```python
from build123d import *

# Parameters (mm, degrees)
SKETCH1_W           = 10
SKETCH1_H           = 8
BOSS_EXTRUDE1_DEPTH = 10.9
CHAMFER1_SIZE       = 1.35
CHAMFER1_SIZE2      = 4.0347247
SKETCH2_W           = 10
SKETCH2_H           = 3.5
CUT_EXTRUDE1_DEPTH  = 1.35
SKETCH3_W           = 4
SKETCH3_H           = 5
CUT_EXTRUDE2_DEPTH  = 7
CHAMFER2_SIZE       = 1.2
CUT_EXTRUDE3_DEPTH  = 0.65
SKETCH5_R           = 1.9
CUT_EXTRUDE4_DEPTH  = 5.25
BOSS_EXTRUDE3_DEPTH = 7.4
CUT_EXTRUDE5_DEPTH  = 7.2


with BuildPart() as part:
    # Sketch1 → Boss-Extrude1 (new body)
    with BuildSketch(Plane.XY):
        Rectangle(SKETCH1_W, SKETCH1_H)
    extrude(amount=BOSS_EXTRUDE1_DEPTH)

    # Chamfer1
    chamfer1_edges = [part.edges().sort_by_distance(p)[0] for p in [
        (0, -4, 10.9),
    ]]
    chamfer1_side = [part.faces().sort_by_distance(p)[0] for p in [
        (0, 0, 10.9),
    ]]
    chamfer(chamfer1_edges, length=CHAMFER1_SIZE, length2=CHAMFER1_SIZE2, reference=chamfer1_side[0])

    # Sketch2 → Cut-Extrude1 (cut)
    with BuildSketch(Plane(origin=(0, 4, 0), x_dir=(1, 0, 0), z_dir=(0, 1, 0))):
        with Locations((0, -9.15)):
            Rectangle(SKETCH2_W, SKETCH2_H)
    extrude(amount=-CUT_EXTRUDE1_DEPTH, mode=Mode.SUBTRACT)

    # Sketch3 → Cut-Extrude2 (cut)
    with BuildSketch(Plane.XZ.offset(4)):
        with Locations((-2.475, 3.15)):
            Rectangle(SKETCH3_W, SKETCH3_H)
        with Locations((2.475, 3.15)):
            Rectangle(SKETCH3_W, SKETCH3_H)
    extrude(amount=-CUT_EXTRUDE2_DEPTH, mode=Mode.SUBTRACT)

    # Chamfer2
    chamfer2_edges = [part.edges().sort_by_distance(p)[0] for p in [
        (-2.475, -4, 5.65),
        (2.475, -4, 5.65),
    ]]
    chamfer(chamfer2_edges, length=CHAMFER2_SIZE)

    # Sketch4 → Cut-Extrude3 (cut)
    with BuildSketch(Plane(origin=(0, 0, 0), x_dir=(-1, 0, 0), z_dir=(0, 0, -1))):
        Polygon((2, 0.7), (3, 0.7), (3, -2.4), (3.25, -4), (1.75, -4), (2, -2.4), align=None)
        Polygon((-2, 0.7), (-2, -2.4), (-1.75, -4), (-3.25, -4), (-3, -2.4), (-3, 0.7), align=None)
    extrude(amount=-CUT_EXTRUDE3_DEPTH, mode=Mode.SUBTRACT)

    # Sketch5 → Cut-Extrude4 (cut)
    with BuildSketch(Plane.XY.offset(10.9)):
        with Locations((-2.5, 0)):
            Circle(SKETCH5_R)
        with Locations((2.5, 0)):
            Circle(SKETCH5_R)
    extrude(amount=-CUT_EXTRUDE4_DEPTH, mode=Mode.SUBTRACT)

    # Sketch6 → Boss-Extrude3 (add)
    with BuildSketch(Plane(origin=(0, 0, 0), x_dir=(-1, 0, 0), z_dir=(0, 0, -1))):
        Polygon((5, 3.25), (5, 2.85), (5.5, 2.7), (5.5, 3.4), align=None)
    extrude(amount=-BOSS_EXTRUDE3_DEPTH)

    # Sketch7 → Cut-Extrude5 (cut)
    with BuildSketch(Plane(origin=(0, 0, 0), x_dir=(-1, 0, 0), z_dir=(0, 0, -1))):
        Polygon((-5, 3.25), (-4.5, 3.4), (-4.5, 2.7), (-5, 2.85), align=None)
    extrude(amount=-CUT_EXTRUDE5_DEPTH, mode=Mode.SUBTRACT)


solid = part.part
```
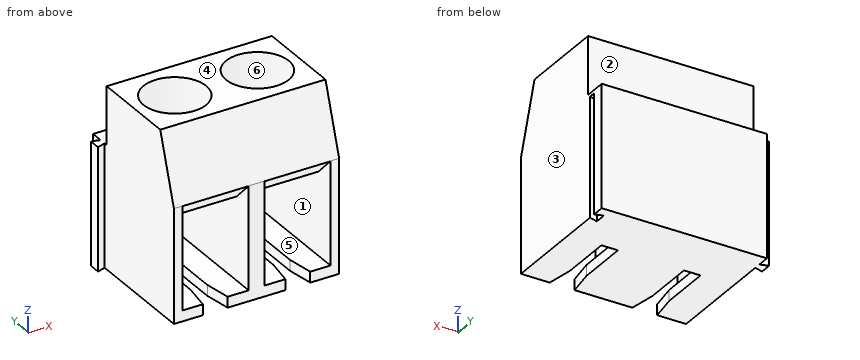
Verification items for the finished model (mm, model axes). Face numbers are marked on the shaded views. A direction names the side the tool comes from. Give positions to 0.01 mm unless a question says otherwise; leave off trailing zeros. Order: outer loops, then holes, each group sorted by start corner. A loop starts at its lowest first (then second) coordinate and runs counter-clockwise, first axis right, second up. Notation, with made-up numbers: (73.25, 26.25) - (82.25, 26.25) arc R11 ccw to (82.25, 36.25) - close; hole circle Ø7 at (30.5, 20). An arc over 180 degrees is marked (long way). Answer as CSV lines item,"result". Start each with the question number.
Item 1: Mould release check, pull along X, two halves, no side actions. Record for the marked faces 1, 2 and 3: released by +X, released by -X, zero draft, split by the parting line, or undercut.
Item 2: Section check B-B, the plane z = 6. Record the boundary of the cut face in (x, y) (3 decimals).
Item 3: Material ranges on L1, parallel to X at y = -1.25, z = 4 (3 decimals); L2, parallel to X at y = -0.75, z = 9; L3, parallel to Z at x = -3.75, y = 2.75, recorded low to high.
Item 4: Gauge pin test, flat ends, axial feed: pin 1 (0.8 mm diameter, centred on y = 3.5, z = 4, fed in from -X); pin 2 (1 mm diameter, centred on y = -1.5, z = 1, fed in from -X); pin 3 (0.5 mm diameter, centred on x = 2.5, z = 0, fed in from -Y); pin 4 (1.8 mm diameter, centred on x = -1.5, z = 10, fed in from +Y). Record the tip position at first contact, or that the pin passes through.
Item 5: Section check D-D, the plane z = 2.5. Record the boundary of the cut face in (x, y) (3 decimals), plus the area to 3 significant figures.
Item 6: Section check C-C, the plane y = 0. Record the boundary of the cut face in (x, z) (3 decimals), plus the area to 3 significant figures.
Item 7: Access from +Z, -Z, +X, -X, +Y, -Y to the whole of each face (thin tool, end or side, straight path). Record for the marked faces 4, 5 and 6.
Filled in:
1,face 1,"undercut"
1,face 2,"zero draft"
1,face 3,"released by +X"
2,outline,"(-5.5, 2.7) - (-5, 2.85) - (-5, -4) - (-4.475, -4) - (-4.475, -3.15) - (-0.475, -3.15) - (-0.475, -4) - (0.475, -4) - (0.475, -3.15) - (4.475, -3.15) - (4.475, -4) - (5, -4) - (5, 2.85) - (4.5, 2.7) - (4.5, 3.4) - (5, 3.25) - (5, 4) - (-5, 4) - (-5, 3.25) - (-5.5, 3.4) - close; hole circle Ø3.8 at (-2.5, 0); hole circle Ø3.8 at (2.5, 0)"
3,L1,"-5 to -4.475, -0.475 to 0.475, 4.475 to 5"
3,L2,"-5 to -4.25, -0.75 to 0.75, 4.25 to 5"
3,L3,"0 to 0.65, 5.65 to 7.4"
4,pin 1,"x = -5.5"
4,pin 2,"x = -5"
4,pin 3,"y = 0.7"
4,pin 4,"y = 2.65"
5,outline,"(-5.5, 2.7) - (-5, 2.85) - (-5, -4) - (-4.475, -4) - (-4.475, 3) - (-0.475, 3) - (-0.475, -4) - (0.475, -4) - (0.475, 3) - (4.475, 3) - (4.475, -4) - (5, -4) - (5, 2.85) - (4.5, 2.7) - (4.5, 3.4) - (5, 3.25) - (5, 4) - (-5, 4) - (-5, 3.25) - (-5.5, 3.4) - close"
5,area,"24.0 mm^2"
6,outline,"(-5, 0) - (-3, 0) - (-3, 0.65) - (-4.475, 0.65) - (-4.475, 5.65) - (-4.4, 5.65) - (-4.4, 10.9) - (-5, 10.9) - close; (-2, 0) - (2, 0) - (2, 0.65) - (0.475, 0.65) - (0.475, 5.65) - (0.6, 5.65) - (0.6, 10.9) - (-0.6, 10.9) - (-0.6, 5.65) - (-0.475, 5.65) - (-0.475, 0.65) - (-2, 0.65) - close; (3, 0) - (5, 0) - (5, 10.9) - (4.4, 10.9) - (4.4, 5.65) - (4.475, 5.65) - (4.475, 0.65) - (3, 0.65) - close"
6,area,"27.8 mm^2"
7,face 4,"+Z, +X, -X, +Y, -Y"
7,face 5,"-Y"
7,face 6,"+Z"
